CAD build for the part. Positions are in the model's coordinates, mm. Give positions to 0.01 mm unless a question says otherwise; leave off trailing zeros. Order: outer loops, then holes, each group sorted by start corner. A loop starts at its lowest first (then second) coordinate and runs counter-clockwise, first axis right, second up.
Autodesk Fusion 360 part; units mm, degrees
sketch "Schizzo1" plane through (0, 0, 0) normal (0, 0, 1) x (1, 0, 0)
  line L0 (-50, 0) -> (7.5, 0)
  line L1 (-49.5, 37) -> (-50, 0)
  line L2 (7, 37) -> (7.5, 0)
  line L3 (-49.5, 37) -> (7, 37)
  dimension "d7" = 57.5
extrude "Estrusione1" add sketch "Schizzo1" along normal blind 1.4
fillet "Raccordo1" radius 2 4 edges at (-50, 0, 0.7) (-49.5, 37, 0.7) (7, 37, 0.7) (7.5, 0, 0.7)
sketch "Schizzo2" plane through (0, 0, 1.4) normal (0, 0, 1) x (-1, 0, 0)
  line L0 (47.9728, 0) -> (-5.4728, 0)
  line L1 (-7.4726, -2.027) -> (-7.0267, -35.027)
  line L2 (-5.0268, -37) -> (47.5268, -37)
  line L3 (49.5267, -35.027) -> (49.9726, -2.027)
  arc A0 (-5.4728, 0) -> (-7.4726, -2.027) centre (-5.4728, -2) ccw
  arc A1 (-7.0267, -35.027) -> (-5.0268, -37) centre (-5.0268, -35) ccw
  arc A2 (47.5268, -37) -> (49.5267, -35.027) centre (47.5268, -35) ccw
  arc A3 (49.9726, -2.027) -> (47.9728, 0) centre (47.9728, -2) ccw
  line L4 (-5.4728, -2) -> (48, -2)
  line L5 (48, -2) -> (48, -3)
  line L6 (48, -3) -> (-5.4728, -3)
  line L7 (-5.4728, -3) -> (-5.4728, -2)
extrude "Estrusione2" add sketch "Schizzo2" along normal blind 0.5 contours L4 L5 L6 L7
fillet "Raccordo2" radius 0.5 4 edges at (-21.2636, 3, 1.9) (-21.2636, 2, 1.9) (5.4728, 2.5, 1.9) (-48, 2.5, 1.9)
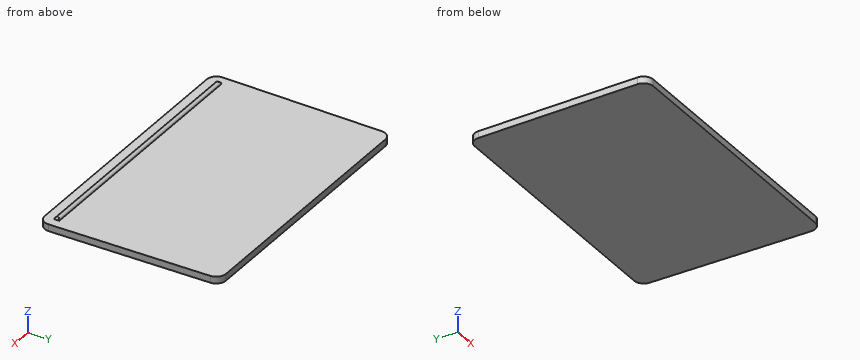
1. Pin check, flat tips, straight feed: P1, Ø2, axis at x = -26, y = 8.5, coming from the +Z side; P2, Ø1, axis at y = 27.5, z = 1.5, coming from the -X side (3 decimals). Stop position of each tip, or through.
2. Saw through at C-C on y = 29. Give the cut face in (x, z), plus the area to 3 significant figures.
3. Saw through at B-B on y = 24.5. Give the cut face in (x, z), plus the area to 3 significant figures.
4. Wall check: line 1 (Z direction, x = -34, y = 16.5); line 2 (Y direction, x = -20, z = 1.6); line 3 (X direction, y = 23.5, z = 1.3). Give the ranges that are in metal, low to high.
Reported:
1. P1: stops at z = 1.4
1. P2: stops at x = -49.635
2. outline: (-49.61, 0) - (7.11, 0) - (7.11, 1.4) - (-49.61, 1.4) - close
2. area: 79.4 mm2
3. outline: (-49.67, 0) - (7.17, 0) - (7.17, 1.4) - (-49.67, 1.4) - close
3. area: 79.6 mm2
4. line 1: z = 0 to 1.4
4. line 2: y = 2.04 to 2.96
4. line 3: x = -49.68 to 7.18
